```python
from build123d import *

# Parameters (mm, degrees)
ESQUISSE1_R             = 2
ESQUISSE1_R_2           = 1.8
BOSS_EXTRU_1_DEPTH      = 2
ESQUISSE3_R             = 3.5
ENL_V_MAT_EXTRU_1_DEPTH = 0.5
CHANFREIN1_SIZE         = 0.5


with BuildPart() as part:
    # Esquisse1 → Boss.-Extru.1 (new body)
    with BuildSketch(Plane.XY):
        with BuildLine():
            Line((0, 0), (0, 20))
            add(Edge.make_bspline(
                [(0, 20), (8, 20), (39, 10), (70, 15), (80, 15)],
                knots=[0, 0, 0, 0, 0, 1, 1, 1, 1, 1], degree=4))
            Line((80, 15), (80, 5))
            add(Edge.make_bspline(
                [(0, 0), (8, 0), (39, 10), (70, 5), (80, 5)],
                knots=[0, 0, 0, 0, 0, 1, 1, 1, 1, 1], degree=4))
        make_face()
        with Locations((3.85, 15)):
            Circle(ESQUISSE1_R, mode=Mode.SUBTRACT)
        with Locations((3.85, 5)):
            Circle(ESQUISSE1_R, mode=Mode.SUBTRACT)
        with Locations((57, 10)):
            Circle(ESQUISSE1_R_2, mode=Mode.SUBTRACT)
        with Locations((75, 10)):
            Circle(ESQUISSE1_R_2, mode=Mode.SUBTRACT)
        with Locations((20, 10)):
            Circle(ESQUISSE1_R_2, mode=Mode.SUBTRACT)
        with Locations((40, 10)):
            Circle(ESQUISSE1_R_2, mode=Mode.SUBTRACT)
    extrude(amount=BOSS_EXTRU_1_DEPTH)

    # Esquisse3 → Enlèv. mat.-Extru.1 (cut)
    with BuildSketch(Plane.XY.offset(2)):
        with Locations((57, 10)):
            Circle(ESQUISSE3_R)
        with Locations((75, 10)):
            Circle(ESQUISSE3_R)
    extrude(amount=-ENL_V_MAT_EXTRU_1_DEPTH, mode=Mode.SUBTRACT)

    # Chanfrein1
    chanfrein1_edges = [part.edges().sort_by_distance(p)[0] for p in [
        (55.2, 10, 1.5),
        (73.2, 10, 1.5),
    ]]
    chamfer(chanfrein1_edges, length=CHANFREIN1_SIZE)


solid = part.part
```
The model under review builds one solid part; all positions refer to its coordinate system, in mm. A direction names the side the tool comes from. Round coordinates to 2 decimals unless told otherwise and drop trailing zeros.
(1) Machinability: for faces 1 (the cylindrical face through (78.233, 8.659, 1.754)), 2 (the cylindrical face through (3.59, 16.983, 0.986)), which of the approach directions +Z, -Z, +X, -X, +Y, -Y give a long, thin tool a straight path to every point of the face, cutting with its end or side? Answer none if there is none.
(2) Wall thickness on L1, parallel to Y at x = 57, z = 0.35; L2, parallel to Y at x = 5, z = 1.2; L3, parallel to Y at x = 4, z = 0.5: over which ranges is each line inside the solid? List them lowest first.
(3) We need section A-A on y = 10. Give the number of separate pieces and of enclosed holes in the cut face, and give its area (3 significant figures).
(4) Insertion check: pin 1 (3.5 mm diameter, centred on x = 3.85, y = 15, fed in from -Z); pin 2 (3.5 mm diameter, centred on x = 55.5, y = 9.5, fed in from +Z). Each pin has a flat end and moves straight along its axis. Give the tip position at first contact, or say it passes through.
(5) Mouldability with a two-part tool opening along Y and no side actions: class faces 3 (the flat face through (32, 10, 2)), 4 (the cylindrical face through (3.59, 6.983, 0.986)) as +Y half, -Y half, draft (parallel to the pull), parting line (faces both ways), or undercut.
Findings below:
1. face 1: +Z
1. face 2: +Z, -Z
2. L1: y = 5.92 to 8.2, 11.8 to 14.08
2. L2: y = 0.59 to 3.36, 6.64 to 13.36, 16.64 to 19.41
2. L3: y = 0.43 to 3.01, 6.99 to 13.01, 16.99 to 19.57
3. separate pieces: 5
3. enclosed holes: 0
3. area: 127 mm2
4. pin 1: passes through
4. pin 2: stops at z = 1.5
5. face 3: draft
5. face 4: undercut
